Could you check a few things on this model? Use its own coordinates, in mm. A direction names the side the tool comes from. Coordinates: 2 decimals unless noted, no trailing zeros. Loops run counter-clockwise (first coordinate to the right, second up) from the corner with the lowest first, then second, coordinate; pieces in that order, holes last. Notation, with made-up numbers: (66.25, 60.5) - (115.25, 60.5) arc R19 cw to (115.25, 92.5) - close; hole circle Ø2 at (89, 87). An arc over 180 degrees is marked (long way). Use CSV: the item, a comma, the result in double quotes.
from build123d import *

# Parameters (mm, degrees)
SKETCH1_R           = 11
BOSS_EXTRUDE1_DEPTH = 25
SKETCH2_R           = 10
BOSS_EXTRUDE2_DEPTH = 2
SKETCH3_R           = 1
BOSS_EXTRUDE3_DEPTH = 5


with BuildPart() as part:
    # Sketch1 → Boss-Extrude1 (new body)
    with BuildSketch(Plane(origin=(0, 0, 0), x_dir=(0, 0, -1), z_dir=(1, 0, 0))):
        Circle(SKETCH1_R)
    extrude(amount=BOSS_EXTRUDE1_DEPTH)

    # Sketch2 → Boss-Extrude2 (add)
    with BuildSketch(Plane(origin=(25, 0, 0), x_dir=(0, 0, -1), z_dir=(1, 0, 0))):
        Circle(SKETCH2_R)
    extrude(amount=BOSS_EXTRUDE2_DEPTH)

    # Sketch3 → Boss-Extrude3 (add)
    with BuildSketch(Plane(origin=(27, 0, 0), x_dir=(0, 0, -1), z_dir=(1, 0, 0))):
        Circle(SKETCH3_R)
    extrude(amount=BOSS_EXTRUDE3_DEPTH)


solid = part.part
(1) Suppose I cut it at D-D (z = 4.75). Write out the boundary of the cut face in (x, y), plus the area to 3 significant figures.
Computed:
outline,"(0, -9.92) - (25, -9.92) - (25, -8.8) - (27, -8.8) - (27, 8.8) - (25, 8.8) - (25, 9.92) - (0, 9.92) - close"
area,"531 mm²"
(2) Which directions (+Z, -Z, +X, -X, +Y, -Y) give clear straight access to the entire face, cutting with the end or side of a thin tool? Please do faces 1 (the face through (25, -10, -2)), 2 (the face through (12.32, -10.74, 2.38)).
Computed:
face 1,"+X"
face 2,"+X, -X"
(3) Suppose I cut it at A-A (y = 0). Write out the boundary of the cut face in (x, z), plus the area to 3 significant figures.
Computed:
outline,"(0, -11) - (25, -11) - (25, -10) - (27, -10) - (27, -1) - (32, -1) - (32, 1) - (27, 1) - (27, 10) - (25, 10) - (25, 11) - (0, 11) - close"
area,"600 mm²"
(4) Please list where these lines run through material, in increasing order: line 1 (X direction, y = -5.5, z = 2); line 2 (X direction, y = -9.5, z = -3.5); line 3 (Z direction, x = 5.5, y = -0.25).
Computed:
line 1,"x = 0 to 27"
line 2,"x = 0 to 25"
line 3,"z = -11 to 11"
(5) Suppose I cut it at C-C (x = 28). Write out the boundary of the cut face in (y, z).
Computed:
outline,"circle Ø2 at (0, 0)"
(6) Will these pins go through, and if not, where does the flat tip stop? pin 1 (1 mm diameter, centred on x = 21.5, z = 7.5, fed in from -Y); pin 2 (6 mm diameter, centred on x = 16, y = -4, fed in from +Z); pin 3 (3 mm diameter, centred on y = 3.5, z = -5.5, fed in from +X).
Computed:
pin 1,"stops at y = -8.49"
pin 2,"stops at z = 10.95"
pin 3,"stops at x = 27"
